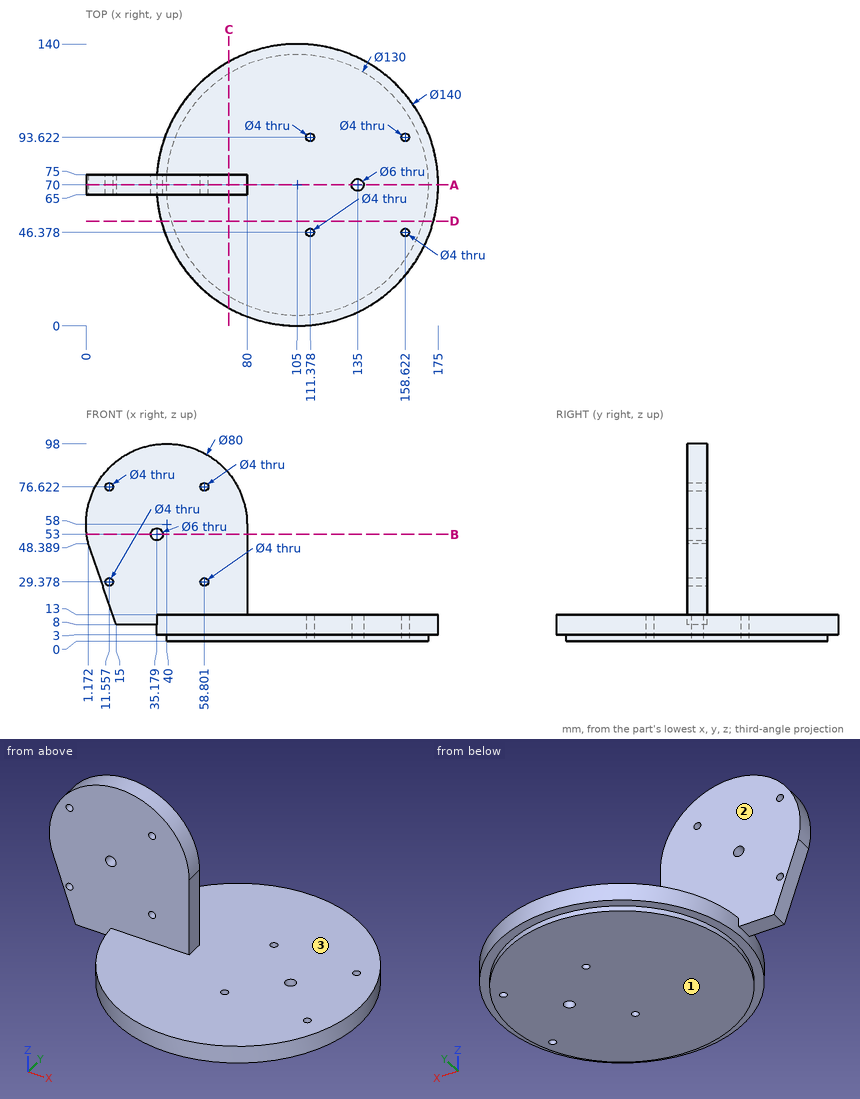
Could you check a few things on this drawing? It's one solid part, dimensions in mm from its lowest x, y, z. Coordinates: 2 decimals unless noted, no trailing zeros. Order: outer loops, then holes, each group sorted by start corner. A loop starts at its lowest first (then second) coordinate and runs counter-clockwise, first axis right, second up. Notation, with made-up numbers: (82.5, -21) -> (140.5, -21) arc R29 ccw to (140.5, -1) -> close; hole circle Ø4 at (79.5, -2.5). An arc over 180 degrees is marked (long way). Answer in a Markdown table with one row per item.
(1) I want a section at D-D on y = 52. List the corners of the cut face in (x, z) for me, then the cut area to 3 significant figures.
Answer key:
| item | result |
|---|---|
| outline | (37.35, 3) -> (42.54, 3) -> (42.54, 0) -> (167.46, 0) -> (167.46, 3) -> (172.65, 3) -> (172.65, 13) -> (37.35, 13) -> close |
| area | 1,730 mm^2 |
(2) Will these pins go through, and if not, where does the flat tip stop? pin 1 Ø6.5 at (x, y) = (158.62, 46.38) entering from -Z; pin 2 Ø10 at (x, z) = (79, 15) entering from -Y; pin 3 Ø11 at (x, y) = (28, 69) entering from -Z; pin 4 Ø8 at (y, z) = (67.5, 26) entering from +X.
Answer key:
| item | result |
|---|---|
| pin 1 | z = 0 |
| pin 2 | y = 3.36 |
| pin 3 | z = 8 |
| pin 4 | x = 80 |
(3) Thinking about a two-plate mould opening in Z: for the marked faces 1, 2 and 3, which applies, +Z half, -Z half, draft (parallel to the pull), parting line (faces both ways), or undercut?
Answer key:
| item | result |
|---|---|
| face 1 | -Z half |
| face 2 | draft |
| face 3 | +Z half |
(4) I want a section at C-C on x = 71. List the corners of the cut face in (y, z) for me, then the cut area to 3 significant figures.
Answer key:
| item | result |
|---|---|
| outline | (8.81, 3) -> (14.6, 3) -> (14.6, 0) -> (125.4, 0) -> (125.4, 3) -> (131.19, 3) -> (131.19, 13) -> (75, 13) -> (75, 83.28) -> (65, 83.28) -> (65, 13) -> (8.81, 13) -> close |
| area | 2,260 mm^2 |
(5) I want a section at B-B on z = 53. List the corners of the cut face in (x, y) for me, then the cut area to 3 significant figures.
Answer key:
| item | result |
|---|---|
| outline | (0.31, 65) -> (32.18, 65) -> (32.18, 75) -> (0.31, 75) -> close; (38.18, 65) -> (80, 65) -> (80, 75) -> (38.18, 75) -> close |
| area | 737 mm^2 |
(6) I want a section at A-A on y = 70. List the corners of the cut face in (x, z) for me, then the cut area to 3 significant figures.
Answer key:
| item | result |
|---|---|
| outline | (1.17, 48.39) -> (15, 8) -> (35, 8) -> (35, 3) -> (40, 3) -> (40, 0) -> (132, 0) -> (132, 13) -> (80, 13) -> (80, 58) arc R40 ccw (long way) to start; (138, 0) -> (170, 0) -> (170, 3) -> (175, 3) -> (175, 13) -> (138, 13) -> close; hole circle Ø4 at (11.56, 29.38); hole circle Ø4 at (11.56, 76.62); hole circle Ø6 at (35.18, 53); hole circle Ø4 at (58.8, 29.38); hole circle Ø4 at (58.8, 76.62) |
| area | 7,590 mm^2 |
(7) Please list where these lines run through material, in increasing order: probe 1 along X at (y, z) = (70, 6); probe 2 along Z at (x, y) = (145, 35); probe 3 along Y at (x, z) = (18, 28.5).
Answer key:
| item | result |
|---|---|
| probe 1 | 35 to 132, 138 to 175 |
| probe 2 | 0 to 13 |
| probe 3 | 65 to 75 |
